```python
from build123d import *

# Parameters (mm, degrees)
F0_R      = 7.6454
F1_DEPTH  = 53.086
F4_DEPTH  = 15.5204
F5_R      = 3.96875
F6_DEPTH  = 22.225
F7_R      = 2.0828
F8_DEPTH  = 7.62
F9_R      = 1.0922
F10_DEPTH = 7.874
F12_R     = 2.7813
F13_DEPTH = 15.5204
F14_R     = 1.2192
F15_DEPTH = 15.5204


with BuildPart() as f1:
    # F0 (on Right) → F1 (new body)
    with BuildSketch(Plane.YZ):
        Circle(F0_R)
    extrude(amount=-F1_DEPTH)

    # F3 (on offset) → F4 (cut, through all)
    with BuildSketch(Plane.XY.offset(7.874)):
        with BuildLine():
            Line((25.4, 3.5306), (-21.8694, 3.5306))
            ThreePointArc((-21.8694, 3.5306), (-24.365911, 2.496511), (-25.4, 0))
            ThreePointArc((-25.4, 0), (-24.365911, -2.496511), (-21.8694, -3.5306))
            Line((-21.8694, -3.5306), (25.4, -3.5306))
            Line((25.4, -3.5306), (25.4, 3.5306))
        make_face()
    extrude(amount=-F4_DEPTH, mode=Mode.SUBTRACT)

    # F5 (on face) → F6 (cut)
    with BuildSketch(Plane(origin=(-53.086, 0, 0), x_dir=(0, -1, 0), z_dir=(-1, 0, 0))):
        Circle(F5_R)
    extrude(amount=-F6_DEPTH, mode=Mode.SUBTRACT)

    # F7 (on offset) → F8 (cut)
    with BuildSketch(Plane.XY.offset(7.874)):
        with Locations((-46.736, 0)):
            Circle(F7_R)
    extrude(amount=-F8_DEPTH, mode=Mode.SUBTRACT)

    # F9 (on face) → F10 (cut)
    with BuildSketch(Plane.YZ):
        with Locations((5.4356, 0)):
            Circle(F9_R)
    extrude(amount=-F10_DEPTH, mode=Mode.SUBTRACT)

    # F12 (on offset) → F13 (cut, through all)
    with BuildSketch(Plane.XZ.offset(7.874)):
        with Locations((-15.875, 0)):
            Circle(F12_R)
    extrude(amount=-F13_DEPTH, mode=Mode.SUBTRACT)

    # F14 (on offset) → F15 (cut, through all)
    with BuildSketch(Plane.XZ.offset(7.874)):
        with Locations((-37.211, 0)):
            Circle(F14_R)
    extrude(amount=-F15_DEPTH, mode=Mode.SUBTRACT)


solid = f1.part
```
The model under review builds one solid part; all positions refer to its coordinate system, in mm. A direction names the side the tool comes from. Give positions to 0.01 mm unless a question says otherwise; leave off trailing zeros. Loops run counter-clockwise (first coordinate to the right, second up) from the corner with the lowest first, then second, coordinate; pieces in that order, holes last. Notation, with made-up numbers: (-37, 31.25) - (-30, 31.25) arc R15 cw to (-30, 37.25) - close; hole circle Ø9 at (13, 77). An arc over 180 degrees is marked (long way). Answer as a JSON object with one key per item and string values.
Q1. Add section B-B on y = -0.5. State the section outline as (x, z) points.
Worked out:
{"outline": "(-53.09, -7.63) - (-25.36, -7.63) - (-25.36, 7.63) - (-44.71, 7.63) - (-44.71, 3.94) - (-30.86, 3.94) - (-30.86, -3.94) - (-53.09, -3.94) - close; (-53.09, 3.94) - (-48.76, 3.94) - (-48.76, 7.63) - (-53.09, 7.63) - close"}
Q2. Insertion check: pin 1 (8.5 mm diameter, centred on y = -1, z = -0.5, fed in from -X); pin 2 (1.3 mm diameter, centred on y = 5.44, z = 0, fed in from +X); pin 3 (4.5 mm diameter, centred on x = -15.875, z = 0, fed in from -Y); pin 4 (6 mm diameter, centred on x = -31.5, z = -5.5, fed in from +Y). Each pin has a flat end and moves straight along its axis. Give the tip position at first contact, or say it passes through.
Worked out:
{"pin 1": "stops at x = -53.09", "pin 2": "stops at x = -7.87", "pin 3": "passes through", "pin 4": "stops at y = 7.23"}
Q3. To check wall thickness, follow line 1 along X through (y, z) = (-5, 0); line 2 along X through (y, z) = (4.8, 0); line 3 along Y through (x, z) = (-47, 2). State the ranges of each line that lie inside material, in increasing order.
Worked out:
{"line 1": "x = -53.09 to -38.43, -35.99 to -18.66, -13.09 to 0", "line 2": "x = -53.09 to -38.43, -35.99 to -18.66, -13.09 to -7.87", "line 3": "y = -7.38 to -3.43, 3.43 to 7.38"}
Q4. Add section D-D on z = 2.25. State the section outline as (x, y) points.
Worked out:
{"outline": "(-53.09, -7.31) - (-17.51, -7.31) - (-17.51, -3.53) - (-21.87, -3.53) arc R3.53 cw to (-25.4, 0) arc R3.53 cw to (-21.87, 3.53) - (-17.51, 3.53) - (-17.51, 7.31) - (-53.09, 7.31) - (-53.09, 3.27) - (-30.86, 3.27) - (-30.86, -3.27) - (-53.09, -3.27) - close; (-14.24, -7.31) - (0, -7.31) - (0, -3.53) - (-14.24, -3.53) - close; (-14.24, 3.53) - (0, 3.53) - (0, 7.31) - (-14.24, 7.31) - close"}
Q5. For faces 1 (the cylindrical face through (-18.654, 5.559, 0.122)), 2 (the cylindrical face through (-3.882, 6.477, 0.328)), 3 (the flat face through (-11, 3.531, 0)), 4 (the cylindrical face through (-26.17, -1, 7.58)), 5 (the flat face through (-30.861, 0, 0)), list the 3-axis set-ups (+Z, -Z, +X, -X, +Y, -Y) from which the entire face can be reached by the end or side of a thin tool; tool diameter is ignored.
Worked out:
{"face 1": "+Y, -Y", "face 2": "+X", "face 3": "+Z, -Z, +X", "face 4": "+X, -X", "face 5": "-X"}
Q6. Mouldability with a two-part tool opening along X and no side actions: class faces 6 (the flat face through (-11, -3.531, 0)), 7 (the flat face through (-7.874, 5, 0)), 8 (the cylindrical face through (-48.817, 0.092, 5.546)) as +X half, -X half, draft (parallel to the pull), parting line (faces both ways), or undercut.
Worked out:
{"face 6": "draft", "face 7": "+X half", "face 8": "undercut"}
Q7. Add section C-C on x = -14. State the section outline as (y, z) points, plus the area to 3 significant figures.
Worked out:
{"outline": "(-7.36, -2.05) arc R7.65 ccw to (-3.53, -6.78) - (-3.53, -2.05) - close; (-7.36, 2.05) - (-3.53, 2.05) - (-3.53, 6.78) arc R7.65 ccw to start; (3.53, -6.78) arc R7.65 ccw to (7.36, -2.05) - (3.53, -2.05) - close; (3.53, 2.05) - (7.36, 2.05) arc R7.65 ccw to (3.53, 6.78) - close", "area": "46.6 mm^2"}
Q8. Add section A-A on z = 0. Count the separate pieces of the cut face and the enclosed holes in it, plus the area to 3 significant figures.
Worked out:
{"separate pieces": "5", "enclosed holes": "0", "area": "380 mm^2"}
